Work out the finished part from the listing and answer in its coordinate system (mm). Give positions to 0.01 mm unless a question says otherwise; leave off trailing zeros. Loops run counter-clockwise (first coordinate to the right, second up) from the corner with the lowest first, then second, coordinate; pieces in that order, holes last. Notation, with made-up numbers: (75, 1) - (80, 1) arc R22 ccw to (80, 25) - close; hole circle Ø6 at (-28, 12). An arc over 180 degrees is marked (long way). One line per item, written item: value.
Autodesk Inventor part; units mm, degrees
ref_plane "YZ Plane" through (0, 0, 0) normal (1, 0, 0) x (0, 1, 0)
ref_plane "XZ Plane" through (0, 0, 0) normal (0, 1, 0) x (-1, 0, 0)
ref_plane "XY Plane" through (0, 0, 0) normal (0, 0, 1) x (1, 0, 0)
sketch "Sketch1" plane through (0, 0, 0) normal (0, 1, 0) x (-1, 0, 0)
  circle A0 centre (0, 0) radius 44.45
  dimension "d0" = 88.9
extrude "Extrusion1" add sketch "Sketch1" along normal blind 50.8
sketch "Sketch2" plane through (0, 0, 0) normal (0, -1, 0) x (1, 0, 0)
  circle A0 centre (0, 0) radius 25.4
  dimension "d3" = 50.8
extrude "Extrusion2" add sketch "Sketch2" along normal blind 50.8
loft "Loft1" add section 1 edges at (-25.4, -50.8, 0) section 2 edges at (44.45, 0, 0)
properties part number "Thing2"
1. Find the intervals of material crossed by line 1 along Z through (x, y) = (-28.5, -23); line 2 along X through (y, z) = (12.5, -19.5); line 3 along X through (y, z) = (22, 2), in increasing order.
Output:
line 1: z = -21.71 to 21.71
line 2: x = -39.94 to 39.94
line 3: x = -44.4 to 44.4
2. Section C-C (y = -33) is taken. Write down the section's boundary in (x, z) (3 decimals).
Output:
outline: circle Ø64.15 at (0, 0)
3. Flat-ended cylindrical pins translate along their axes: pin 1 Ø3 at (y, z) = (20.5, -32) entering from +X (3 decimals); pin 2 Ø12 at (y, z) = (-36, 27) entering from -X; pin 3 Ø1.5 at (x, y) = (18, 36) entering from +Z. Find the tip coordinate at first contact, or state that the pin passes through.
Output:
pin 1: stops at x = 32.335
pin 2: stops at x = -23.53
pin 3: stops at z = 40.97
4. Section A-A (x = 0) is taken. Write down the section's boundary in (y, z), and give its area (3 significant figures).
Output:
outline: (-50.8, -25.4) - (0, -44.45) - (50.8, -44.45) - (50.8, 44.45) - (0, 44.45) - (-50.8, 25.4) - close
area: 8,060 mm²
5. Section B-B (y = 14.5) is taken. Write down the section's boundary in (x, z).
Output:
outline: circle Ø88.9 at (0, 0)
